Check sheet for the modelled part. Datum: model origin and axes. Units: mm. A direction names the side the tool comes from. Round coordinates to 2 decimals unless told otherwise and drop trailing zeros. Loops run counter-clockwise (first coordinate to the right, second up) from the corner with the lowest first, then second, coordinate; pieces in that order, holes last. Notation, with made-up numbers: (10.25, 50) - (28.25, 50) arc R25 cw to (28.25, 72) - close; hole circle Ø8 at (81.25, -25). An arc over 180 degrees is marked (long way). Return JSON: item names as keys, results as strings.
from build123d import *

# Parameters (mm, degrees)
CHAMFER1_SIZE           = 0.762
CUT_EXTRUDE1_DEPTH      = 256.026625277
CUT_EXTRUDE1_DEPTH_BACK = 256.026625277
SKETCH2_W               = 9.652
SKETCH2_H               = 20.7772
SKETCH3_R               = 3.9624
CUT_EXTRUDE2_DEPTH      = 256.026625277


with BuildPart() as part:
    # Sketch1 → Revolve1 (revolve)
    with BuildSketch(Plane(origin=(0, 0, 0), x_dir=(0, 0, -1), z_dir=(1, 0, 0)), mode=Mode.PRIVATE) as revolve1_sk:
        with BuildLine():
            Line((0, 8.7376), (0, 22.225))
            Line((0, 22.225), (203.2, 22.225))
            Line((203.2, 22.225), (215.644604414, 41.950024019))
            ThreePointArc((215.644604414, 41.950024019), (216.962465562, 48.723970202), (213.36, 54.61))
            Line((213.36, 54.61), (213.36, 76.2))
            Line((213.36, 76.2), (231.14, 76.2))
            Line((231.14, 76.2), (231.14, 54.61))
            Line((231.14, 54.61), (217.150682631, 32.43656548))
            ThreePointArc((217.150682631, 32.43656548), (215.740333448, 26.296391433), (218.471224769, 20.618975231))
            Line((218.471224769, 20.618975231), (223.2152, 15.875))
            Line((223.2152, 15.875), (223.2152, 8.7376))
            Line((223.2152, 8.7376), (0, 8.7376))
        make_face()
    revolve(revolve1_sk.sketch.rotate(Axis((0, 0, 0), (0, 0, -1)), 90), axis=Axis((0, 0, 0), (0, 0, -1)))

    # Chamfer1
    chamfer1_edges = [part.edges().sort_by_distance(p)[0] for p in [
        (-76.2, 0, -231.14),
        (-76.2, 0, -213.36),
    ]]
    chamfer(chamfer1_edges, length=CHAMFER1_SIZE)

    # Sketch2 → Cut-Extrude1 (cut, two sides: drawn at the far end of the back side and taken through both)
    with BuildSketch(Plane(origin=(0, 0, 0), x_dir=(0, 0, -1), z_dir=(1, 0, 0)).offset(-CUT_EXTRUDE1_DEPTH_BACK)):
        with Locations((4.826, 0)):
            Rectangle(SKETCH2_W, SKETCH2_H)
    extrude(amount=CUT_EXTRUDE1_DEPTH + CUT_EXTRUDE1_DEPTH_BACK, mode=Mode.SUBTRACT)

    # Sketch3 → Cut-Extrude2 (cut, through all)
    with BuildSketch(Plane(origin=(0, 0, -231.14), x_dir=(-1, 0, 0), z_dir=(0, 0, -1))):
        with Locations((0, 65.405)):
            Circle(SKETCH3_R)
    extrude(amount=-CUT_EXTRUDE2_DEPTH, mode=Mode.SUBTRACT)


solid = part.part
Q1. Depth check by flat-ended pin: P1, Ø10.5, axis at x = 0, y = 65.405, coming from the +Z side; P2, Ø9.5, axis at x = -3.5, y = 0, coming from the -Z side (1 decimal); P3, Ø6, axis at x = -8, z = -190, coming from the +Y side; P4, Ø10.5, axis at x = -3.5, y = -5, coming from the +Z side. Enter the tip coordinate at first touch or a pass-through.
Answer key:
{"P1": "stops at z = -213.36", "P2": "passes through", "P3": "stops at y = 21.66", "P4": "stops at z = -9.65"}
Q2. Sectioned sample at C-C (z = -96). Enter the section's corners in (x, y) (3 decimals).
Answer key:
{"outline": "circle Ø44.45 at (0, 0); hole circle Ø17.475 at (0, 0)"}
Q3. Sectioned sample at A-A (y = 0). Enter the section's corners in (x, z) (3 decimals).
Answer key:
{"outline": "(-76.2, -230.378) - (-75.438, -231.14) - (-54.61, -231.14) - (-32.437, -217.151) arc R9.525 cw to (-20.619, -218.471) - (-15.875, -223.215) - (-8.738, -223.215) - (-8.738, -9.652) - (-22.225, -9.652) - (-22.225, -203.2) - (-41.95, -215.645) arc R9.525 cw to (-54.61, -213.36) - (-75.438, -213.36) - (-76.2, -214.122) - close; (8.738, -223.215) - (15.875, -223.215) - (20.619, -218.471) arc R9.525 cw to (32.437, -217.151) - (54.61, -231.14) - (75.438, -231.14) - (76.2, -230.378) - (76.2, -214.122) - (75.438, -213.36) - (54.61, -213.36) arc R9.525 cw to (41.95, -215.645) - (22.225, -203.2) - (22.225, -9.652) - (8.738, -9.652) - close"}
Q4. Scan lines: probe 1 along Y at (x, z) = (0, -89) (3 decimals); probe 2 along Y at (x, z) = (13.5, -218); probe 3 along Y at (x, z) = (0, -226). Record each from-to range of solid material in increasing order. Write a range as [from, to].
Answer key:
{"probe 1": "y = [-22.225, -8.738], [8.738, 22.225]", "probe 2": "y = [-74.99, -30.97], [-16.25, 16.25], [30.97, 74.99]", "probe 3": "y = [-76.2, -46.46], [46.46, 61.44], [69.37, 76.2]"}
Q5. Draft check along Y on faces 4 (the face through (-16.519, 74.388, -222.364)), 5 (the face through (39, -39, -231.14)), 6 (the face through (8.334, -2.625, -114.939)), 7 (the face through (7, 7, -223.215)). Enter one of: released by +Y, released by -Y, zero draft, split by the parting line, or undercut.
Answer key:
{"face 4": "split by the parting line", "face 5": "zero draft", "face 6": "undercut", "face 7": "undercut"}
Q6. Tool access check on faces 1 (the face through (-16.4, -15, -103)), 2 (the face through (0, 15, 0)), 3 (the face through (0, 10.389, -5)). Record the directions out of +Z, -Z, +X, -X, +Y, -Y that give a thin tool (end or side, any length) a straight path to the whole face; none if there is none.
Answer key:
{"face 1": "+Z", "face 2": "+Z, +X, -X, +Y, -Y", "face 3": "+Z, +X, -X"}
Q7. Sectioned sample at B-B (x = 0). State how many separate pieces and enclosed holes the cut face has, plus the area to 3 significant figures.
Answer key:
{"separate pieces": "3", "enclosed holes": "0", "area": "7,190 mm²"}
